from build123d import *

# Parameters (mm, degrees)
SKETCH1_W                                  = 700
SKETCH1_H                                  = 700
BOSS_EXTRUDE1_DEPTH                        = 6.35
SKETCH2_W                                  = 155
SKETCH2_H                                  = 55
CUT_EXTRUDE2_DEPTH                         = 10
MIRROR1_AT_THE_SECOND_PLANE_COPY_1_SKETC_W = 155
MIRROR1_AT_THE_SECOND_PLANE_COPY_1_SKETC_H = 55
MIRROR1_AT_THE_SECOND_PLANE_COPY_1_DEPTH   = 10
SKETCH3_W                                  = 10
SKETCH3_H                                  = 20
SKETCH3_W_2                                = 15
CUT_EXTRUDE3_DEPTH                         = 990.96985939


with BuildPart() as part:
    # Sketch1 → Boss-Extrude1 (new body)
    with BuildSketch(Plane(origin=(0, 0, 0), x_dir=(1, 0, 0), z_dir=(0, 1, 0))):
        with Locations((350, 350)):
            Rectangle(SKETCH1_W, SKETCH1_H)
    extrude(amount=BOSS_EXTRUDE1_DEPTH)

    # Sketch2 → Cut-Extrude2 (cut)
    with BuildSketch(Plane(origin=(0, 6.35, 0), x_dir=(1, 0, 0), z_dir=(0, 1, 0))):
        with BuildLine():
            ThreePointArc((572.75, 110), (569.933273811, 111.166726189), (571.1, 108.35))
            Line((571.1, 108.35), (571.1, 110))
            Line((571.1, 110), (572.75, 110))
        make_face()
        with BuildLine():
            Line((571.1, 110), (571.1, 108.35))
            ThreePointArc((571.1, 108.35), (572.266726189, 108.833273811), (572.75, 110))
            Line((572.75, 110), (571.1, 110))
        make_face()
        with BuildLine():
            ThreePointArc((571.1, 101.65), (569.933273811, 98.833273811), (572.75, 100))
            Line((572.75, 100), (571.1, 100))
            Line((571.1, 100), (571.1, 101.65))
        make_face()
        with BuildLine():
            Line((571.1, 100), (572.75, 100))
            ThreePointArc((572.75, 100), (572.266726189, 101.166726189), (571.1, 101.65))
            Line((571.1, 101.65), (571.1, 100))
        make_face()
        with BuildLine():
            ThreePointArc((609.45, 110), (609.933273811, 108.833273811), (611.1, 108.35))
            Line((611.1, 108.35), (611.1, 110))
            Line((611.1, 110), (609.45, 110))
        make_face()
        with BuildLine():
            Line((611.1, 110), (611.1, 108.35))
            ThreePointArc((611.1, 108.35), (612.266726189, 108.833273811), (612.75, 110))
            ThreePointArc((612.75, 110), (611.1, 111.65), (609.45, 110))
            Line((609.45, 110), (611.1, 110))
        make_face()
        with BuildLine():
            ThreePointArc((611.1, 101.65), (609.933273811, 101.166726189), (609.45, 100))
            Line((609.45, 100), (611.1, 100))
            Line((611.1, 100), (611.1, 101.65))
        make_face()
        with BuildLine():
            Line((611.1, 100), (609.45, 100))
            ThreePointArc((609.45, 100), (611.1, 98.35), (612.75, 100))
            ThreePointArc((612.75, 100), (612.266726189, 101.166726189), (611.1, 101.65))
            Line((611.1, 101.65), (611.1, 100))
        make_face()
        with Locations((591.1, 47.5)):
            Rectangle(SKETCH2_W, SKETCH2_H)
    cut_extrude2 = extrude(amount=-CUT_EXTRUDE2_DEPTH, mode=Mode.SUBTRACT)

    # Mirror1: Cut-Extrude2 across plane
    add(cut_extrude2.mirror(Plane(origin=(350, 0, 0), x_dir=(0, 0, 1), z_dir=(1, 0, 0))), mode=Mode.SUBTRACT)

    # Mirror1 at the second plane: Cut-Extrude2 across plane
    add(cut_extrude2.mirror(Plane.XY.offset(-350)), mode=Mode.SUBTRACT)

    # Mirror1 at the second plane copy 1 sketc → Mirror1 at the second plane copy 1 (cut)
    with BuildSketch(Plane(origin=(700, 6.35, -700), x_dir=(-1, 0, 0), z_dir=(0, 1, 0))):
        with BuildLine():
            ThreePointArc((572.75, 110), (569.933273811, 111.166726189), (571.1, 108.35))
            Line((571.1, 108.35), (571.1, 110))
            Line((571.1, 110), (572.75, 110))
        make_face()
        with BuildLine():
            Line((571.1, 110), (571.1, 108.35))
            ThreePointArc((571.1, 108.35), (572.266726189, 108.833273811), (572.75, 110))
            Line((572.75, 110), (571.1, 110))
        make_face()
        with BuildLine():
            ThreePointArc((571.1, 101.65), (569.933273811, 98.833273811), (572.75, 100))
            Line((572.75, 100), (571.1, 100))
            Line((571.1, 100), (571.1, 101.65))
        make_face()
        with BuildLine():
            Line((571.1, 100), (572.75, 100))
            ThreePointArc((572.75, 100), (572.266726189, 101.166726189), (571.1, 101.65))
            Line((571.1, 101.65), (571.1, 100))
        make_face()
        with BuildLine():
            ThreePointArc((609.45, 110), (609.933273811, 108.833273811), (611.1, 108.35))
            Line((611.1, 108.35), (611.1, 110))
            Line((611.1, 110), (609.45, 110))
        make_face()
        with BuildLine():
            Line((611.1, 110), (611.1, 108.35))
            ThreePointArc((611.1, 108.35), (612.266726189, 108.833273811), (612.75, 110))
            ThreePointArc((612.75, 110), (611.1, 111.65), (609.45, 110))
            Line((609.45, 110), (611.1, 110))
        make_face()
        with BuildLine():
            ThreePointArc((611.1, 101.65), (609.933273811, 101.166726189), (609.45, 100))
            Line((609.45, 100), (611.1, 100))
            Line((611.1, 100), (611.1, 101.65))
        make_face()
        with BuildLine():
            Line((611.1, 100), (609.45, 100))
            ThreePointArc((609.45, 100), (611.1, 98.35), (612.75, 100))
            ThreePointArc((612.75, 100), (612.266726189, 101.166726189), (611.1, 101.65))
            Line((611.1, 101.65), (611.1, 100))
        make_face()
        with Locations((591.1, 47.5)):
            Rectangle(MIRROR1_AT_THE_SECOND_PLANE_COPY_1_SKETC_W, MIRROR1_AT_THE_SECOND_PLANE_COPY_1_SKETC_H)
    extrude(amount=-MIRROR1_AT_THE_SECOND_PLANE_COPY_1_DEPTH, mode=Mode.SUBTRACT)

    # Sketch3 → Cut-Extrude3 (cut, through all)
    with BuildSketch(Plane(origin=(0, 6.35, 0), x_dir=(1, 0, 0), z_dir=(0, 1, 0))):
        with Locations((567.5, 315)):
            Rectangle(SKETCH3_W, SKETCH3_H)
        with Locations((602.5, 315)):
            Rectangle(SKETCH3_W, SKETCH3_H)
        with Locations((537.5, 250)):
            Rectangle(SKETCH3_W_2, SKETCH3_H)
        with Locations((632.5, 250)):
            Rectangle(SKETCH3_W_2, SKETCH3_H)
        with Locations((567.5, 185)):
            Rectangle(SKETCH3_W, SKETCH3_H)
        with Locations((602.5, 185)):
            Rectangle(SKETCH3_W, SKETCH3_H)
    extrude(amount=-CUT_EXTRUDE3_DEPTH, mode=Mode.SUBTRACT)


solid = part.part
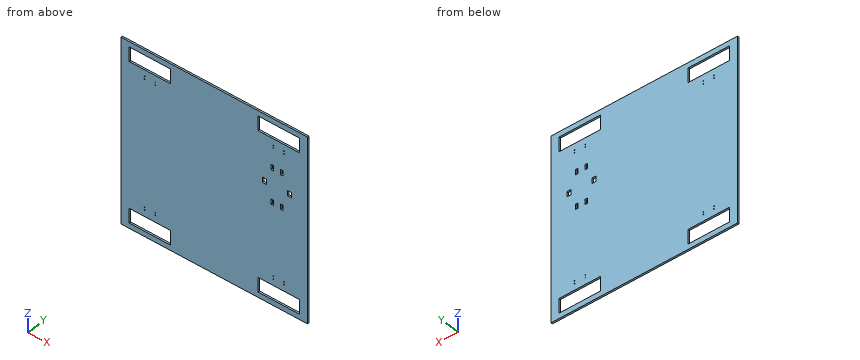
Could you check a few things on this model? Use its own coordinates, in mm. Round coordinates to 2 decimals unless told otherwise and drop trailing zeros. Use a Markdown table: item, result.
Q1. Please list where these lines run through material, in increasing order: L1, parallel to Z at x = 116, y = 5.75; L2, parallel to X at y = 2.75, z = -590; L3, parallel to Z at x = 637, y = 1.5.
Output values:
| item | result |
|---|---|
| L1 | -700 to -680, -625 to -75, -20 to 0 |
| L2 | 0 to 87.25, 90.55 to 127.25, 130.55 to 569.45, 572.75 to 609.45, 612.75 to 700 |
| L3 | -700 to -680, -625 to -260, -240 to -75, -20 to 0 |
Q2. For pin 1 (3 mm diameter, centred on x = 321, y = 2.5, fed in from +Z), with a flat end and sliding along its axis, tell me the tip position at first contact or that it passes through.
Output values:
| item | result |
|---|---|
| pin 1 | z = 0 |
Q3. I want a section at A-A (y = 2.75). Count the separate pieces of the cut face and the enclosed holes in it, plus the area to 3 significant figures.
Output values:
| item | result |
|---|---|
| separate pieces | 1 |
| enclosed holes | 26 |
| area | 454,000 mm2 |
